Design review of the part built by this model. Coordinates are the model's own, in mm. Face numbers are marked on the shaded views. A direction names the side the tool comes from. Round coordinates to 2 decimals unless told otherwise and drop trailing zeros. Order: outer loops, then holes, each group sorted by start corner. A loop starts at its lowest first (then second) coordinate and runs counter-clockwise, first axis right, second up. Notation, with made-up numbers: (54.25, 2.25) - (61.25, 2.25) arc R17 ccw to (61.25, 10.25) - close; hole circle Ø10 at (-2, -28.5). An arc over 180 degrees is marked (long way). Write item = value, one per line.
from build123d import *

# Parameters (mm, degrees)
SKETCH1_W           = 25.4
SKETCH1_H           = 25.4
BOSS_EXTRUDE1_DEPTH = 7.62
BOSS_EXTRUDE2_DEPTH = 5.08
SKETCH3_R           = 5.053169443
CUT_EXTRUDE1_DEPTH  = 26.4


with BuildPart() as part:
    # Sketch1 → Boss-Extrude1 (new body)
    with BuildSketch(Plane(origin=(0, 0, 0), x_dir=(1, 0, 0), z_dir=(0, 1, 0))):
        Rectangle(SKETCH1_W, SKETCH1_H)
    extrude(amount=BOSS_EXTRUDE1_DEPTH)

    # Sketch2 → Boss-Extrude2 (add)
    with BuildSketch(Plane(origin=(12.7, 0, 0), x_dir=(0, 0, -1), z_dir=(1, 0, 0))):
        with BuildLine():
            Line((-12.7, 7.62), (-9.412998127, 19.887257994))
            ThreePointArc((-9.412998127, 19.887257994), (0, 24.05658338), (9.412998127, 19.887257994))
            Line((9.412998127, 19.887257994), (12.7, 7.62))
            Line((12.7, 7.62), (-12.7, 7.62))
        make_face()
    boss_extrude2 = extrude(amount=-BOSS_EXTRUDE2_DEPTH)

    # Mirror1: Boss-Extrude2 across plane
    add(boss_extrude2.mirror(Plane(origin=(0, 0, 0), x_dir=(0, 0, 1), z_dir=(1, 0, 0))))

    # Sketch3 → Cut-Extrude1 (cut, through all)
    with BuildSketch(Plane(origin=(12.7, 0, 0), x_dir=(0, 0, -1), z_dir=(1, 0, 0))):
        with Locations((0, 13.97)):
            Circle(SKETCH3_R)
    extrude(amount=-CUT_EXTRUDE1_DEPTH, mode=Mode.SUBTRACT)


solid = part.part
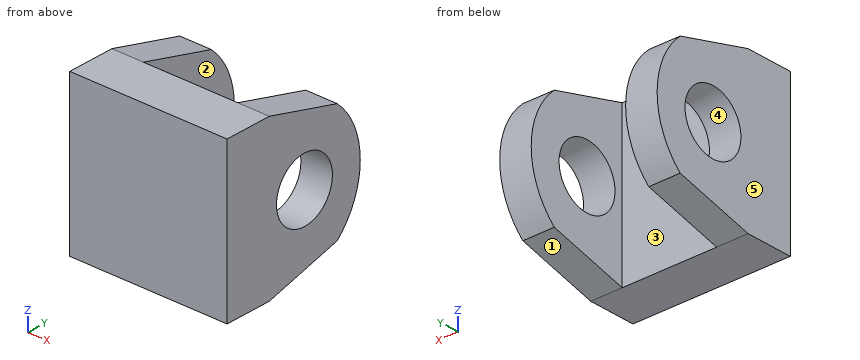
1) Clearance check with flat-ended pins moving along their axes: pin 1 Ø9 at (y, z) = (13.97, 0) entering from -X; pin 2 Ø5 at (x, z) = (8.5, -5.5) entering from +Y. State where each tip first meets the part, or that it passes through.
Findings:
pin_1 = through
pin_2 = 23.7
2) We need section D-D on z = -7.25. Write out the cut boundary in (x, y), and give its area (3 significant figures).
Findings:
outline = (-12.7, 0) - (12.7, 0) - (12.7, 21.79) - (7.62, 21.79) - (7.62, 7.62) - (-7.62, 7.62) - (-7.62, 21.79) - (-12.7, 21.79) - close
area = 337 mm^2
3) For the marked faces 1 and 2, list the 3-axis set-ups (+Z, -Z, +X, -X, +Y, -Y) from which the entire face can be reached by the end or side of a thin tool; tool diameter is ignored.
Findings:
face_1 = -Z, +X, -X, +Y
face_2 = +Z, -Z, +Y
4) We need section A-A on z = 0. Write out the cut boundary in (x, y), and give its area (3 significant figures).
Findings:
outline = (-12.7, 0) - (12.7, 0) - (12.7, 8.92) - (7.62, 8.92) - (7.62, 7.62) - (-7.62, 7.62) - (-7.62, 8.92) - (-12.7, 8.92) - close; (-12.7, 19.02) - (-7.62, 19.02) - (-7.62, 24.06) - (-12.7, 24.06) - close; (7.62, 19.02) - (12.7, 19.02) - (12.7, 24.06) - (7.62, 24.06) - close
area = 258 mm^2
5) We need section B-B on x = 8. Write out the cut boundary in (y, z).
Findings:
outline = (0, -12.7) - (7.62, -12.7) - (19.89, -9.41) arc R12.71 ccw to (19.89, 9.41) - (7.62, 12.7) - (0, 12.7) - close; hole circle Ø10.11 at (13.97, 0)
6) To check wall thickness, follow L1, parallel to X at y = 17.5, z = 7.5; L2, parallel to Y at x = -10, z = 0; L3, parallel to Y at x = -2.25, z = -6.75. State the ranges of each line that lie inside material, in increasing order. Write a range as from..to.
Findings:
L1 = -12.7..-7.62, 7.62..12.7
L2 = 0..8.92, 19.02..24.06
L3 = 0..7.62
7) We need section C-C on y = 17. Write out the cut boundary in (x, z).
Findings:
outline = (-12.7, -10.19) - (-7.62, -10.19) - (-7.62, -4.04) - (-12.7, -4.04) - close; (-12.7, 4.04) - (-7.62, 4.04) - (-7.62, 10.19) - (-12.7, 10.19) - close; (7.62, -10.19) - (12.7, -10.19) - (12.7, -4.04) - (7.62, -4.04) - close; (7.62, 4.04) - (12.7, 4.04) - (12.7, 10.19) - (7.62, 10.19) - close
8) The part is to be moulded in two halves that separate along X. For the marked faces 3, 4 and 5, say which applies: released by +X, released by -X, zero draft, split by the parting line, or undercut.
Findings:
face_3 = undercut
face_4 = zero draft
face_5 = released by -X
